Here's how the part is built. I have some questions about the finished solid (model axes, mm). Face numbers are marked on the shaded views. A direction names the side the tool comes from. Give positions to 0.01 mm unless a question says otherwise; leave off trailing zeros. Loops run counter-clockwise (first coordinate to the right, second up) from the corner with the lowest first, then second, coordinate; pieces in that order, holes last. Notation, with made-up numbers: (59.5, -25.75) - (79.5, -25.75) arc R18 ccw to (79.5, -19.75) - close; hole circle Ø3 at (-18.75, 63). An arc over 180 degrees is marked (long way). Use one line per item in the form item = value.
from build123d import *

# Parameters (mm, degrees)
F0_W      = 98.6741781235
F0_H      = 41.0901270807
F1_DEPTH  = 19.558
F2_R      = 9.1792961358
F2_R_2    = 9.5503911514
F3_DEPTH  = 38.354
F4_W      = 55.3103350103
F4_H      = 22.0765508711
F5_DEPTH  = 17.526
F6_W      = 21.1468022317
F6_H      = 22.0765508711
F7_DEPTH  = 5.08
F9_DEPTH  = 159.766
F11_DEPTH = 17.018
F13_DEPTH = 17.272
F14_R     = 4.5299196653
F15_DEPTH = 118.872


with BuildPart() as f1:
    # F0 (on Top) → F1 (new body)
    with BuildSketch(Plane.XY):
        Rectangle(F0_W, F0_H)
        with BuildLine():
            ThreePointArc((49.3370890617, -20.5450635403), (69.8821526021, 0), (49.3370890617, 20.5450635403))
            Line((49.3370890617, 20.5450635403), (49.3370890617, -20.5450635403))
        make_face()
        with BuildLine():
            Line((-49.3370890617, -20.5450635403), (-49.3370890617, 20.5450635403))
            ThreePointArc((-49.3370890617, 20.5450635403), (-69.8821526021, 0), (-49.3370890617, -20.5450635403))
        make_face()
    extrude(amount=F1_DEPTH)

    # F2 (on face) → F3 (cut)
    with BuildSketch(Plane.XY.offset(19.558)):
        with Locations((49.3370890617, 0)):
            Circle(F2_R)
        with Locations((-49.3370890617, 0)):
            Circle(F2_R_2)
    extrude(amount=-F3_DEPTH, mode=Mode.SUBTRACT)

    # F4 (on face) → F5 (join)
    with BuildSketch(Plane.XY.offset(19.558)):
        Rectangle(F4_W, F4_H)
    extrude(amount=F5_DEPTH)

    # F6 (on face) → F7 (cut)
    with BuildSketch(Plane.XY.offset(37.084)):
        Rectangle(F6_W, F6_H)
    extrude(amount=-F7_DEPTH, mode=Mode.SUBTRACT)

    # F8 (on face) → F9 (cut)
    with BuildSketch(Plane(origin=(0, 11.0382754356, 0), x_dir=(-1, 0, 0), z_dir=(0, 1, 0))):
        with BuildLine():
            Line((10.5734011158, 32.004), (-10.5734011158, 32.004))
            ThreePointArc((-10.5734011158, 32.004), (0, 21.4305988842), (10.5734011158, 32.004))
        make_face()
    extrude(amount=-F9_DEPTH, mode=Mode.SUBTRACT)

    # F10 (on face) → F11 (join)
    with BuildSketch(Plane.YZ.offset(27.6551675051)):
        with BuildLine():
            Line((-11.0382754356, 37.084), (11.0382754356, 37.084))
            ThreePointArc((11.0382754356, 37.084), (0, 48.1222754356), (-11.0382754356, 37.084))
        make_face()
    extrude(amount=-F11_DEPTH)

    # F12 (on face) → F13 (join)
    with BuildSketch(Plane(origin=(-27.6551675051, 0, 0), x_dir=(0, -1, 0), z_dir=(-1, 0, 0))):
        with BuildLine():
            Line((-11.0382754356, 37.084), (11.0382754356, 37.084))
            ThreePointArc((11.0382754356, 37.084), (0, 48.1222754356), (-11.0382754356, 37.084))
        make_face()
    extrude(amount=-F13_DEPTH)

    # F14 (on face) → F15 (cut)
    with BuildSketch(Plane.YZ.offset(27.6551675051)):
        with Locations((0, 37.084)):
            Circle(F14_R)
    extrude(amount=-F15_DEPTH, mode=Mode.SUBTRACT)


solid = f1.part
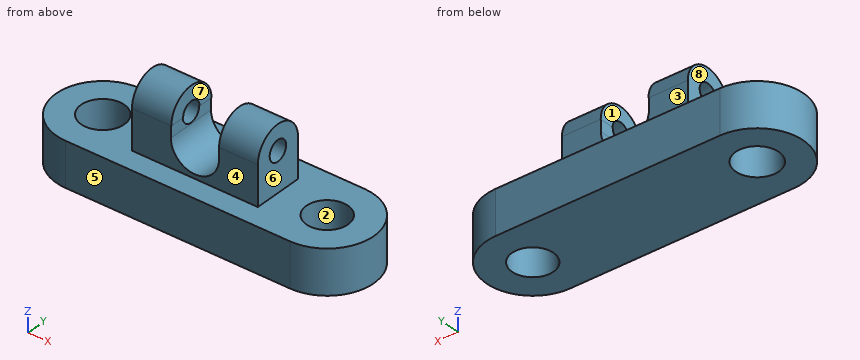
(1) If we section it at A-A (y = 0): List the corners of the cut face in (x, z) for me.
Geometry says:
outline = (-69.88, 0) - (-58.89, 0) - (-58.89, 19.56) - (-69.88, 19.56) - close; (-39.79, 0) - (40.16, 0) - (40.16, 19.56) - (27.66, 19.56) - (27.66, 32.55) - (10.57, 32.55) - (10.57, 32) arc R10.57 cw to (-10.57, 32) - (-10.57, 32.55) - (-27.66, 32.55) - (-27.66, 19.56) - (-39.79, 19.56) - close; (-27.66, 41.61) - (-10.38, 41.61) - (-10.38, 48.12) - (-27.66, 48.12) - close; (10.64, 41.61) - (27.66, 41.61) - (27.66, 48.12) - (10.64, 48.12) - close; (58.52, 0) - (69.88, 0) - (69.88, 19.56) - (58.52, 19.56) - close
(2) If we section it at C-C (z = 6.5): List the corners of the cut face in (x, y) for me.
Geometry says:
outline = (-49.34, -20.55) - (49.34, -20.55) arc R20.55 ccw to (49.34, 20.55) - (-49.34, 20.55) arc R20.55 ccw to start; hole circle Ø19.1 at (-49.34, 0); hole circle Ø18.36 at (49.34, 0)
(3) For P1, Ø11, axis at y = 0, z = 30, coming from the +X side; P2, Ø3.5, axis at y = 5, z = 44, coming from the -X side; P3, Ø4, axis at y = -16, z = 21, coming from the +X side, each with a flat end and sliding along its axis, tell me the tip position at first contact or that it passes through.
Geometry says:
P1 = 27.66
P2 = -27.66
P3 = 63.78
(4) Thinking about a two-plate mould opening in X: for the marked faces 6, 7 and 8, which applies, pulls with the +X half, pulls with the -X half, needs draft (parallel to the pull), parting line crosses it, or undercut?
Geometry says:
face_6 = pulls with the +X half
face_7 = undercut
face_8 = pulls with the -X half
(5) If we section it at B-B (x = 25.5): List the corners of the cut face in (y, z) for me, plus the area to 3 significant figures.
Geometry says:
outline = (-20.55, 0) - (20.55, 0) - (20.55, 19.56) - (11.04, 19.56) - (11.04, 37.08) arc R11.04 ccw to (-11.04, 37.08) - (-11.04, 19.56) - (-20.55, 19.56) - close; hole circle Ø9.06 at (0, 37.08)
area = 1,320 mm²
(6) For the marked faces 1, 2, 3, 4 and 5, which set-ups out of +Z, -Z, +X, -X, +Y, -Y let a thin tool reach every point of the face, with its end or its side?
Geometry says:
face_1 = +Z, +Y, -Y
face_2 = +Z, -Z
face_3 = +Z, +X, -X, +Y
face_4 = +Z, +X, -X, -Y
face_5 = +Z, -Z, +X, -X, -Y
(7) If we section it at D-D (x = 0): List the corners of the cut face in (y, z) for me.
Geometry says:
outline = (-20.55, 0) - (20.55, 0) - (20.55, 19.56) - (11.04, 19.56) - (11.04, 21.43) - (-11.04, 21.43) - (-11.04, 19.56) - (-20.55, 19.56) - close
(8) If I drill on probe 1 along X at (y, z) = (1, 18.5); probe 2 along X at (y, z) = (-10.5, 32); probe 3 along X at (y, z) = (1.5, 13), over which ranges is the centre line in solid material (lowest first)?
Geometry says:
probe_1 = -69.86 to -58.83, -39.84 to 40.21, 58.46 to 69.86
probe_2 = -27.66 to -10.57, 10.57 to 27.66
probe_3 = -69.83 to -58.77, -39.91 to 40.28, 58.39 to 69.83
